Verification items for the finished model (mm, model axes). Round coordinates to 2 decimals unless told otherwise and drop trailing zeros. Write each loop counter-clockwise with the first axis right and the second up, starting at its lowest first coordinate (ties: lowest second). Pieces come first, ordered by that corner, then holes.
Autodesk Inventor part; units mm, degrees
ref_plane "2_1_XY" through (0, 0, 0) normal (0, 0, 1) x (1, 0, 0)
ref_plane "2_1_YZ" through (0, 0, 0) normal (1, 0, 0) x (0, 1, 0)
ref_plane "2_1_ZX" through (0, 0, 0) normal (0, 1, 0) x (0, 0, 1)
sketch "Sketch_1" plane through (0, 0, 0) normal (0, 0, 1) x (1, 0, 0)
  line L0 (5, 0) -> (-5, 0)
  line L1 (-5, 14.5) -> (-5, 6.5)
  line L2 (-5, 6.5) -> (-4.5, 6)
  line L3 (-4.5, 6) -> (4.5, 6)
  line L4 (4.5, 6) -> (5, 6.5)
  line L5 (5, 6.5) -> (5, 14.5)
  line L6 (5, 14.5) -> (4.5, 15)
  line L7 (4.5, 15) -> (-4.5, 15)
  line L8 (-4.5, 15) -> (-5, 14.5)
revolve "Revolution1" add sketch "Sketch_1" angle 180 about axis through (5, 0, 0) along (-1, 0, 0)
sketch "Sketch_2" plane through (0, 0, 0) normal (1, 0, 0) x (0, 1, 0)
  line L0 (-16, 0.75) -> (-16, -0.75)
  line L1 (-16, -0.75) -> (16, -0.75)
  line L2 (16, -0.75) -> (16, 0.75)
  line L3 (16, 0.75) -> (-16, 0.75)
extrude "Extrusion1" cut sketch "Sketch_2" along normal mid plane 10
sketch "Sketch3" plane through (-4.5, -5.9529, -0.75) normal (0, 0, 1) x (1, 0, 0)
  point P0 (4.5, -4.0471)
hole "Hole1" at (0, -10, -0.75) direction (0, 0, -1) diameter 3.242 depth 15 countersink diameter 4 countersink angle 90
sketch "Sketch4" plane through (-4.5, 14.9812, -0.75) normal (0, 0, 1) x (1, 0, 0)
  point P0 (4.5, -4.9812)
hole "Hole2" at (0, 10, -0.75) direction (0, 0, -1) diameter 3.242 depth 15 countersink diameter 4 countersink angle 90
ref_plane "2_1_XY" through (0, 0, 0) normal (0, 0, 1) x (1, 0, 0)
ref_plane "2_1_YZ" through (0, 0, 0) normal (1, 0, 0) x (0, 1, 0)
ref_plane "2_1_ZX" through (0, 0, 0) normal (0, 1, 0) x (0, 0, 1)
properties part number "SSCSP12-10p"
Q1. Depth check by flat-ended pin: P1, Ø3, axis at y = 9.5, z = -12.5, coming from the -X side; P2, Ø3, axis at x = 1, y = 6.5, coming from the -Z side; P3, Ø5, axis at x = 0, y = -10, coming from the -Z side; P4, Ø1.5, axis at x = 1, z = -13.5, coming from the -Y side. Enter the tip coordinate at first touch or a pass-through.
Recorded:
P1: stops at x = -5
P2: stops at z = -14.14
P3: stops at z = -12.99
P4: stops at y = -7.9
Q2. Material ranges on line 1 along X through (y, z) = (10, -5.25); line 2 along Y through (x, z) = (0, -5.25); line 3 along Y through (x, z) = (0, -8), recorded low to high.
Recorded:
line 1: x = -5 to -1.62, 1.62 to 5
line 2: y = -14.05 to -11.62, -8.38 to -2.9, 2.9 to 8.38, 11.62 to 14.05
line 3: y = -12.69 to -11.62, -8.38 to 8.38, 11.62 to 12.69
Q3. Release check for a two-part mould opening along Y. For faces 1 (the cylindrical face through (-0.487, 8.454, -6.864)), 2 (the cylindrical face through (0, 0, -15)), 3 (the flat face through (-5, 0, -8)) record: released by +Y, released by -Y, zero draft, split by the parting line, or undercut.
Recorded:
face 1: undercut
face 2: split by the parting line
face 3: zero draft
Q4. Sectioned sample at A-A (x = 0). Enter the section's corners in (y, z).
Recorded:
outline: (-14.98, -0.75) arc R15 ccw to (-11.62, -9.48) - (-11.62, -1.13) - (-12, -0.75) - close; (-8.38, -12.44) arc R15 ccw to (8.38, -12.44) - (8.38, -1.13) - (8, -0.75) - (5.95, -0.75) arc R6 cw to (-5.95, -0.75) - (-8, -0.75) - (-8.38, -1.13) - close; (11.62, -9.48) arc R15 ccw to (14.98, -0.75) - (12, -0.75) - (11.62, -1.13) - close
Q5. Sectioned sample at B-B (y = 0). Enter the section's corners in (x, z), plus the area to 3 significant figures.
Recorded:
outline: (-5, -14.5) - (-4.5, -15) - (4.5, -15) - (5, -14.5) - (5, -6.5) - (4.5, -6) - (-4.5, -6) - (-5, -6.5) - close
area: 89.5 mm2
Q6. Sectioned sample at C-C (x = 3.5). Enter the section's corners in (y, z).
Recorded:
outline: (-14.98, -0.75) arc R15 ccw to (14.98, -0.75) - (5.95, -0.75) arc R6 cw to (-5.95, -0.75) - close
